from build123d import *

# Parameters (mm, degrees)
F0_W     = 1270
F0_H     = 508
F1_DEPTH = 25.4
F2_W     = 76.2
F2_H     = 76.2
F4_W     = 76.2
F4_H     = 76.2


with BuildPart() as f1:
    # F0 (on Top) → F1 (new body)
    with BuildSketch(Plane.XY):
        Rectangle(F0_W, F0_H)
    extrude(amount=F1_DEPTH)

    # F2 (on face) → F5 section 0
    with BuildSketch(Plane(origin=(0, 0, 0), x_dir=(1, 0, 0), z_dir=(0, 0, -1))):
        with Locations((-406.4, 215.9)):
            Rectangle(F2_W, F2_H)
    # F4 (on offset) → F5 section 1
    with BuildSketch(Plane(origin=(0, 0, -390.525), x_dir=(1, 0, 0), z_dir=(0, 0, -1))):
        with Locations((406.4, 215.9)):
            Rectangle(F4_W, F4_H)
    loft()

    # F2 (on face) → F6 section 0
    with BuildSketch(Plane(origin=(0, 0, 0), x_dir=(1, 0, 0), z_dir=(0, 0, -1))):
        with Locations((-406.4, -215.9)):
            Rectangle(F2_W, F2_H)
    # F4 (on offset) → F6 section 1
    with BuildSketch(Plane(origin=(0, 0, -390.525), x_dir=(1, 0, 0), z_dir=(0, 0, -1))):
        with Locations((406.4, -215.9)):
            Rectangle(F4_W, F4_H)
    loft()

    # F2 (on face) → F7 section 0
    with BuildSketch(Plane(origin=(0, 0, 0), x_dir=(1, 0, 0), z_dir=(0, 0, -1))):
        with Locations((406.4, -215.9)):
            Rectangle(F2_W, F2_H)
    # F4 (on offset) → F7 section 1
    with BuildSketch(Plane(origin=(0, 0, -390.525), x_dir=(1, 0, 0), z_dir=(0, 0, -1))):
        with Locations((-406.4, -215.9)):
            Rectangle(F4_W, F4_H)
    loft()

    # F2 (on face) → F8 section 0
    with BuildSketch(Plane(origin=(0, 0, 0), x_dir=(1, 0, 0), z_dir=(0, 0, -1))):
        with Locations((406.4, 215.9)):
            Rectangle(F2_W, F2_H)
    # F4 (on offset) → F8 section 1
    with BuildSketch(Plane(origin=(0, 0, -390.525), x_dir=(1, 0, 0), z_dir=(0, 0, -1))):
        with Locations((-406.4, 215.9)):
            Rectangle(F4_W, F4_H)
    loft()


solid = f1.part
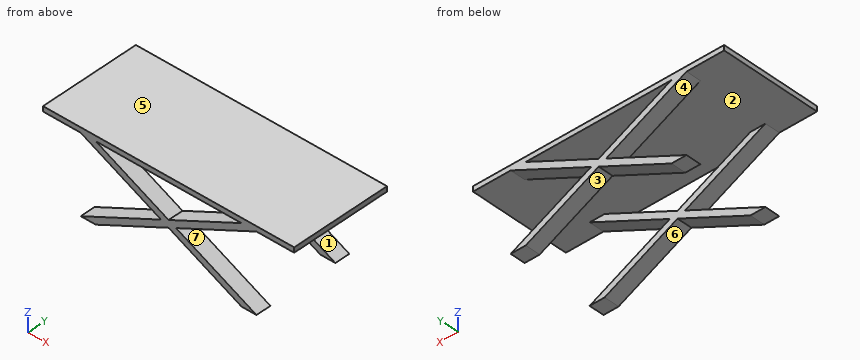
Could you check a few things on this model? Use its own coordinates, in mm. Face numbers are marked on the shaded views. A direction names the side the tool comes from. Give positions to 0.01 mm unless a question says otherwise; leave off trailing zeros. Order: outer loops, then holes, each group sorted by start corner. A loop starts at its lowest first (then second) coordinate and runs counter-clockwise, first axis right, second up.
Item 1: If we section it at A-A, the plane z = -87: Write out the boundary of the cut face in (x, y), plus the area to 3 significant figures.
Item 2: If we section it at B-B, the plane y = 196: Write out the boundary of the cut face in (x, z) (1 decimal).
Item 3: I'm going to push flat-ended pins straight in: pin 1 (8 mm diameter, centred on x = -217.5, y = -24, fed in from -Z); pin 2 (6 mm diameter, centred on x = -151.5, z = -248, fed in from +Y). Where does each tip first touch, or does it pass through?
Item 4: I need wall thicknesses on line 1 (Z direction, x = -29.5, y = -49); line 2 (Z direction, x = -182, y = 216); line 3 (Y direction, x = 270.5, z = -67.5). Which ranges of each line are inside material? Lowest first, please.
Item 5: For the marked faces 1, 2, 3 and 4, which set-ups out of +Z, -Z, +X, -X, +Y, -Y let a thin tool reach every point of the face, with its end or its side?
Item 6: If we section it at D-D, the plane x = -174: Write out the boundary of the cut face in (y, z).
Item 7: If we mould it in two halves opening along Z, with no side actions, what happens to the marked faces 5, 6 and 7? For each: pulls with the +Z half, pulls with the -Z half, needs draft (parallel to the pull), parting line crosses it, or undercut.
Item 8: If we section it at C-C, the plane x = -19: Write out the boundary of the cut face in (y, z), plus the area to 3 significant figures.
Values:
1. outline: (-263.43, -254) - (-187.23, -254) - (-187.23, -177.8) - (-263.43, -177.8) - close; (-263.43, 177.8) - (-187.23, 177.8) - (-187.23, 254) - (-263.43, 254) - close; (187.23, -254) - (263.43, -254) - (263.43, -177.8) - (187.23, -177.8) - close; (187.23, 177.8) - (263.43, 177.8) - (263.43, 254) - (187.23, 254) - close
1. area: 23,200 mm2
2. outline: (-635, 0) - (-444.5, 0) - (-38.1, -195.3) - (-444.5, -390.5) - (-368.3, -390.5) - (0, -213.6) - (368.3, -390.5) - (444.5, -390.5) - (38.1, -195.3) - (444.5, 0) - (635, 0) - (635, 25.4) - (-635, 25.4) - close; hole (-368.3, 0) - (0, -177) - (368.3, 0) - close
3. pin 1: stops at z = 0
3. pin 2: stops at y = 254
4. line 1: z = 0 to 25.4
4. line 2: z = -301.01 to -264.4, -126.12 to -89.51, 0 to 25.4
4. line 3: y = -254 to -177.8, 177.8 to 254
5. face 1: +X, +Y, -Y
5. face 2: none
5. face 3: -Z, +Y, -Y
5. face 4: -X, +Y, -Y
6. outline: (-254, -297.17) - (-177.8, -297.17) - (-177.8, -260.56) - (-254, -260.56) - close; (-254, -129.97) - (-177.8, -129.97) - (-177.8, -93.36) - (-254, -93.36) - close; (-254, 0) - (254, 0) - (254, 25.4) - (-254, 25.4) - close; (177.8, -297.17) - (254, -297.17) - (254, -260.56) - (177.8, -260.56) - close; (177.8, -129.97) - (254, -129.97) - (254, -93.36) - (177.8, -93.36) - close
7. face 5: pulls with the +Z half
7. face 6: pulls with the -Z half
7. face 7: undercut
8. outline: (-254, -222.7) - (-177.8, -222.7) - (-177.8, -167.83) - (-254, -167.83) - close; (-254, 0) - (254, 0) - (254, 25.4) - (-254, 25.4) - close; (177.8, -222.7) - (254, -222.7) - (254, -167.83) - (177.8, -167.83) - close
8. area: 21,300 mm2
